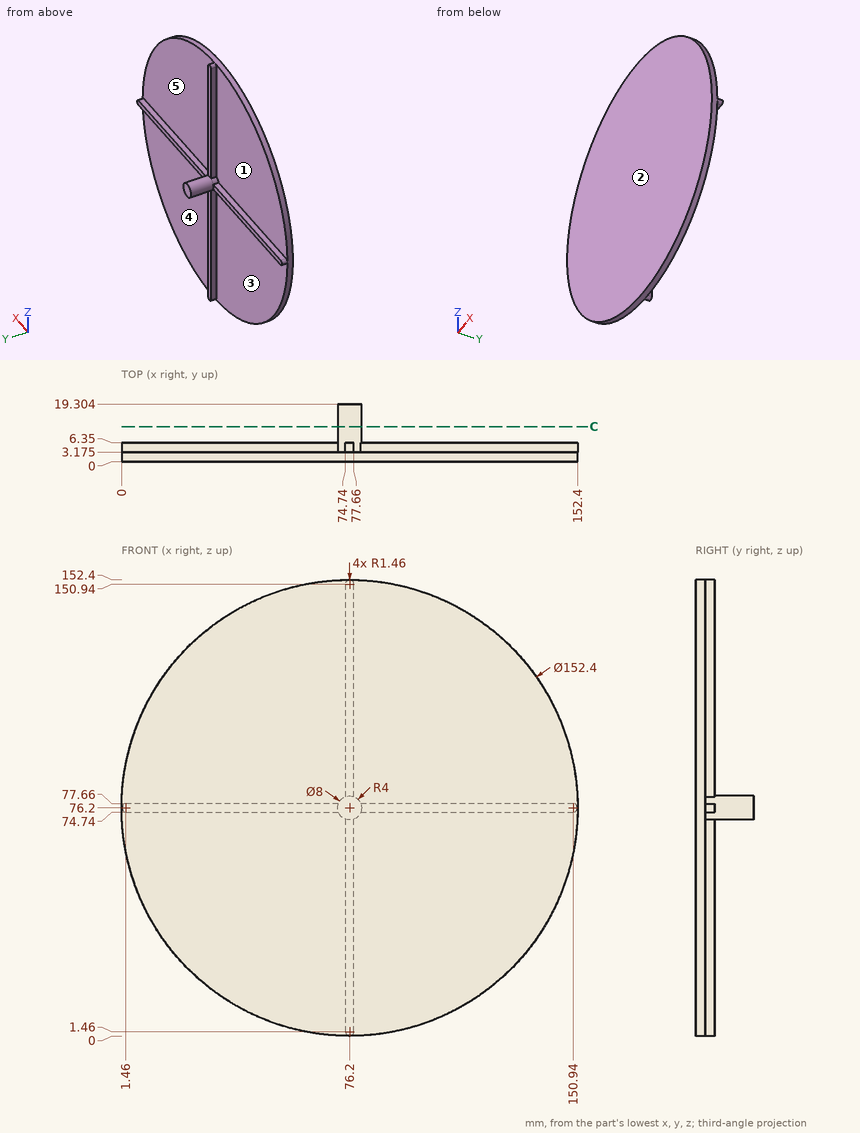
Print and shaded views of the part. All mm, measured from the part's lowest x, y and z. A direction names the side the tool comes from. Coordinates: 2 decimals unless noted, no trailing zeros. Loops run counter-clockwise (first coordinate to the right, second up) from the corner with the lowest first, then second, coordinate; pieces in that order, holes last. Notation, with made-up numbers: (24, 74.5) -> (52, 74.5) arc R23 cw to (52, 104.5) -> close; hole circle Ø10 at (23, 44.5). An arc over 180 degrees is marked (long way). Use a Markdown table: item, result. Add a question column.
Item 1: Probe probe 1 along Y at (x, z) = (48.5, 66.5) (1 decimal); probe 2 along X at (y, z) = (5, 82.5). List the from-to ranges inside material, lowest first.
Item 2: Flat gauge pins, fed straight in: P1, Ø3.5, axis at y = 5.5, z = 104.5, coming from the +X side; P2, Ø2.5, axis at x = 105, y = 4, coming from the -Z side (1 decimal); P3, Ø10, axis at x = 94.5, y = 6.5, coming from the -Z side (1 decimal). Where does each tip first touch, or does it go through?
Item 3: Which spindle directions (+Z, -Z, +X, -X, +Y, -Y) get a long thin tool onto all of the face, cutting with end or side? Do the marked faces 1, 2, 3, 4 and 5. Say none if no direction does.
Item 4: Band-saw the part on C-C on y = 11.75. Write the cut outline in (x, z).
Geometry says:
| question | item | result |
|---|---|---|
| 1 | probe 1 | 0 to 3.2 |
| 1 | probe 2 | 74.74 to 77.66 |
| 2 | P1 | x = 77.66 |
| 2 | P2 | z = 5.3 |
| 2 | P3 | z = 1.4 |
| 3 | face 1 | +Z, -X, +Y |
| 3 | face 2 | +Z, -Z, +X, -X, -Y |
| 3 | face 3 | -Z, -X, +Y |
| 3 | face 4 | -Z, +X, +Y |
| 3 | face 5 | +Z, +X, +Y |
| 4 | outline | circle Ø8 at (76.2, 76.2) |
